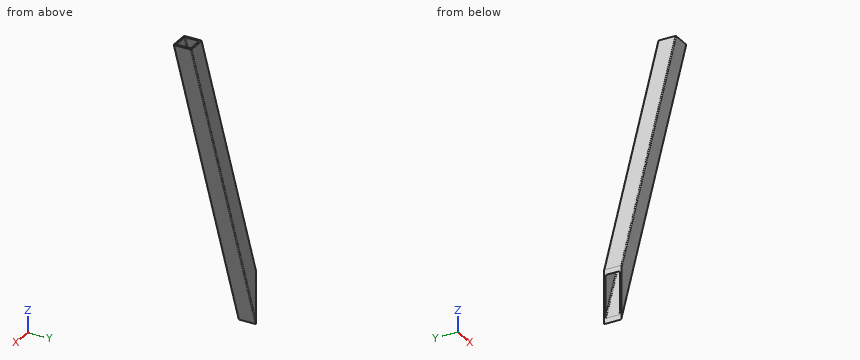
from build123d import *

# Parameters (mm, degrees)
BOSS_EXTRU_1_DEPTH           = 40
COQUE1_T                     = 4
ENL_V_MAT_EXTRU_1_DEPTH      = 833.320761278
ENL_V_MAT_EXTRU_1_DEPTH_BACK = 833.320761278
ESQUISSE2_W                  = 32
ESQUISSE2_H                  = 32
CONG_1_R                     = 2


with BuildPart() as part:
    # Esquisse1 → Boss.-Extru.1 (new body)
    with BuildSketch(Plane(origin=(0, 0, 0), x_dir=(1, 0, 0), z_dir=(0, 1, 0))):
        Polygon((0, 609.961146446), (215.575309292, 0), (258, 0), (0, 730), align=None)
    extrude(amount=BOSS_EXTRU_1_DEPTH)

    # Coque1 (no face opened: a closed hollow body)
    add(offset(amount=-COQUE1_T, mode=Mode.PRIVATE), mode=Mode.SUBTRACT)

    # Esquisse2 → Enlèv. mat.-Extru.1 (cut, two sides: drawn at the far end of the back side and taken through both)
    with BuildSketch(Plane(origin=(23.937308809, 0, 67.729594691), x_dir=(0, -1, 0), z_dir=(-0.33322544172708785, 0, -0.9428471800805194)).offset(-ENL_V_MAT_EXTRU_1_DEPTH_BACK)):
        with Locations((-20, -223.254572461)):
            Rectangle(ESQUISSE2_W, ESQUISSE2_H)
    extrude(amount=ENL_V_MAT_EXTRU_1_DEPTH + ENL_V_MAT_EXTRU_1_DEPTH_BACK, mode=Mode.SUBTRACT)

    # Congé1
    cong_1_edges = [part.edges().sort_by_distance(p)[0] for p in [
        (129, 40, -365),
        (109.908889181, 4, -310.982515901),
        (126.878765465, 4, -358.998057322),
        (109.908889181, 36, -310.982515901),
        (126.878765465, 36, -358.998057322),
        (129, 0, -365),
        (107.787654646, 0, -304.980573223),
        (107.787654646, 40, -304.980573223),
    ]]
    fillet(cong_1_edges, radius=CONG_1_R)


solid = part.part
Here's how the part is built. I have some questions about the finished solid (model axes, mm). Give positions to 0.01 mm unless a question says otherwise; leave off trailing zeros. Order: outer loops, then holes, each group sorted by start corner. A loop starts at its lowest first (then second) coordinate and runs counter-clockwise, first axis right, second up. Notation, with made-up numbers: (-33, 83.5) -> (15, 83.5) arc R9 ccw to (15, 88.5) -> close; hole circle Ø5 at (45, 28.25). An arc over 180 degrees is marked (long way). Use a Markdown table: item, result. Add a question column.
Item 1: Will these pins go through, and if not, where does the flat tip stop? pin 1 (1.5 mm diameter, centred on y = 21, z = -330, fed in from -X); pin 2 (12 mm diameter, centred on y = 5, z = -267.5, fed in from -X); pin 3 (10 mm diameter, centred on y = 25.5, z = -545, fed in from +X).
Item 2: I need wall thicknesses on line 1 (Y direction, x = 155, z = -202.5); line 2 (X direction, y = 17, z = -293.5); line 3 (X direction, y = 13.5, z = -146). Which ranges of each line are inside material? Lowest first, please.
Item 3: Imagine slicing it at A-A on y = 13.5. Please give me the cut outline in (x, z), plus the area to 3 significant figures.
Data:
| question | item | result |
|---|---|---|
| 1 | pin 1 | stops at x = 98.68 |
| 1 | pin 2 | stops at x = 118.91 |
| 1 | pin 3 | stops at x = 67.15 |
| 2 | line 1 | y = 0 to 4, 36 to 40 |
| 2 | line 2 | x = 111.85 to 116.09, 150.03 to 154.27 |
| 2 | line 3 | x = 163.98 to 168.22, 202.16 to 206.4 |
| 3 | outline | (0, -730) -> (258, 0) -> (253.76, 0) -> (0, -718) -> close; (0, -621.97) -> (219.82, 0) -> (215.58, 0) -> (0, -609.96) -> close |
| 3 | area | 5,680 mm² |
